```python
from build123d import *

# Parameters (mm, degrees)
BOSS_EXTRUDE1_DEPTH = 6
SKETCH2_R           = 3
CUT_EXTRUDE1_DEPTH  = 6
CHAMFER2_SIZE       = 1


with BuildPart() as part:
    # Sketch1 → Boss-Extrude1 (new body)
    with BuildSketch(Plane(origin=(0, 0, 0), x_dir=(1, 0, 0), z_dir=(0, 1, 0))):
        Polygon((0, 6.92820323), (-6, 3.464101615), (-6, -3.464101615), (0, -6.92820323), (6, -3.464101615), (6, 3.464101615), align=None)
    extrude(amount=BOSS_EXTRUDE1_DEPTH)

    # Sketch2 → Cut-Extrude1 (cut)
    with BuildSketch(Plane(origin=(0, 6, 0), x_dir=(1, 0, 0), z_dir=(0, 1, 0))):
        Circle(SKETCH2_R)
    extrude(amount=-CUT_EXTRUDE1_DEPTH, mode=Mode.SUBTRACT)

    # Chamfer2
    chamfer2_edges = [part.edges().sort_by_distance(p)[0] for p in [
        (-3, 0, 0),
        (-3, 6, 0),
    ]]
    chamfer(chamfer2_edges, length=CHAMFER2_SIZE)


solid = part.part
```
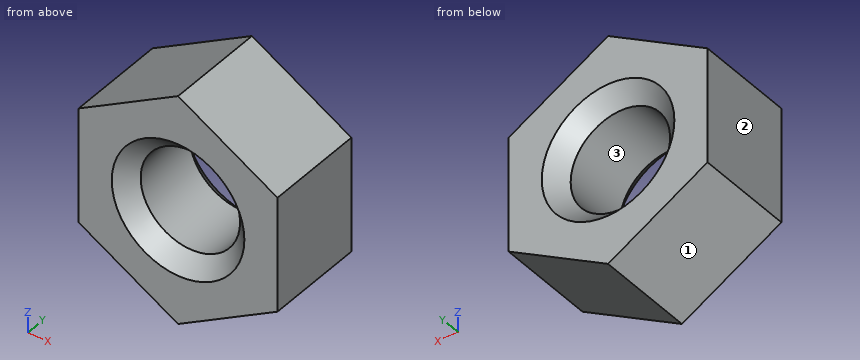
Could you check a few things on this model? Use its own coordinates, in mm. Face numbers are marked on the shaded views. Round coordinates to 2 decimals unless told otherwise and drop trailing zeros. Write each loop counter-clockwise with the first axis right and the second up, starting at its lowest first coordinate (ties: lowest second). Pieces come first, ordered by that corner, then holes.
(1) For pin 1 (3 mm diameter, centred on x = 4.5, y = 4, fed in from -Z); pin 2 (1 mm diameter, centred on x = -3, y = 5, fed in from +Z), each with a flat end and sliding along its axis, tell me the tip position at first contact or that it passes through.
Findings below:
pin 1: stops at z = -5.2
pin 2: stops at z = 5.48
(2) Suppose I cut it at B-B on y = 1.6. Write out the boundary of the cut face in (x, z), and give its area (3 significant figures).
Findings below:
outline: (-6, -3.46) - (0, -6.93) - (6, -3.46) - (6, 3.46) - (0, 6.93) - (-6, 3.46) - close; hole circle Ø6 at (0, 0)
area: 96.4 mm2
(3) If I drill on probe 1 along X at (y, z) = (3.6, 0); probe 2 along Z at (x, y) = (-2, 5.7); probe 3 along X at (y, z) = (5.65, 2.75), over which ranges is the centre line in solid material (lowest first)?
Findings below:
probe 1: x = -6 to -3, 3 to 6
probe 2: z = -5.77 to -3.11, 3.11 to 5.77
probe 3: x = -6 to -2.4, 2.4 to 6
(4) Thinking about a two-plate mould opening in Z: for the marked faces 1, 2 and 3, which applies, +Z half, -Z half, draft (parallel to the pull), parting line (faces both ways), or undercut?
Findings below:
face 1: -Z half
face 2: draft
face 3: undercut
(5) Suppose I cut it at C-C on y = 5.2. Write out the boundary of the cut face in (x, z), and give its area (3 significant figures).
Findings below:
outline: (-6, -3.46) - (0, -6.93) - (6, -3.46) - (6, 3.46) - (0, 6.93) - (-6, 3.46) - close; hole circle Ø6.4 at (0, 0)
area: 92.5 mm2
(6) Suppose I cut it at D-D on x = 5.25. Write out the boundary of the cut face in (y, z).
Findings below:
outline: (0, -3.9) - (6, -3.9) - (6, 3.9) - (0, 3.9) - close
(7) Suppose I cut it at A-A on z = 0. Write out the boundary of the cut face in (x, y), and give its area (3 significant figures).
Findings below:
outline: (-6, 0) - (-4, 0) - (-3, 1) - (-3, 5) - (-4, 6) - (-6, 6) - close; (3, 1) - (4, 0) - (6, 0) - (6, 6) - (4, 6) - (3, 5) - close
area: 34.0 mm2
